from build123d import *

# Parameters (mm, degrees)
BOSS_EXTRUDE2_DEPTH      = 0.79375
FILLET2_R                = 0.396875
CIRPATTERN5_COUNT        = 4
FILLET2_OF_CIRPATTERN5_R = 0.396875
SKETCH6_R                = 10.9855
SKETCH6_R_2              = 9.398
BOSS_EXTRUDE3_DEPTH      = 9.017
SKETCH8_W                = 3.175
SKETCH8_H                = 14.859
SKETCH8_H_2              = 3.175
CUT_EXTRUDE1_DEPTH       = 129.426706448
CUT_EXTRUDE2_REACH       = 130.427
CUT_EXTRUDE2_END_RADIUS  = 10.9855
SKETCH8_3_W              = 3.175
SKETCH8_3_H              = 14.859
SKETCH8_3_H_2            = 3.175


with BuildPart() as part:
    # Sketch3 → Revolve2 (revolve)
    with BuildSketch(Plane(origin=(0, 0, 0), x_dir=(0, 0, -1), z_dir=(1, 0, 0)), mode=Mode.PRIVATE) as revolve2_sk:
        with BuildLine():
            Line((57.15, 12.7), (57.15, 9.525))
            Line((57.15, 9.525), (91.893227671, 9.525))
            ThreePointArc((91.893227671, 9.525), (102.982534669, 8.29739345), (113.534829541, 4.674022024))
            ThreePointArc((113.534829541, 4.674022024), (115.069002319, 4.147228765), (116.68125, 3.96875))
            Line((116.68125, 3.96875), (120.65, 3.96875))
            Line((120.65, 3.96875), (120.65, 3.175))
            Line((120.65, 3.175), (122.2375, 3.175))
            Line((122.2375, 3.175), (125.59178364, 6.52928364))
            Line((125.59178364, 6.52928364), (95.25, 10.32569244))
            ThreePointArc((95.25, 10.32569244), (76.236954553, 12.105847936), (57.15, 12.7))
        make_face()
    revolve(revolve2_sk.sketch.rotate(Axis((0, 0, 0), (0, 0, -1)), 90), axis=Axis((0, 0, 0), (0, 0, -1)))

    # Sketch5 → Boss-Extrude2 (add, symmetric)
    with BuildSketch(Plane(origin=(0, 0, 0), x_dir=(0, 0, -1), z_dir=(1, 0, 0))):
        Polygon((125.59178364, 6.27528364), (95.25, 10.07169244), (119.24178364, 18.97528364), (125.59178364, 18.97528364), align=None)
    boss_extrude2 = extrude(amount=BOSS_EXTRUDE2_DEPTH, both=True)

    # Fillet2
    fillet2_edges = [part.edges().sort_by_distance(p)[0] for p in [
        (0.79375, 18.97528364, -122.41678364),
        (-0.79375, 18.97528364, -122.41678364),
        (0.79375, 14.606978185, -107.47086593),
        (-0.79375, 14.606978185, -107.47086593),
    ]]
    fillet(fillet2_edges, radius=FILLET2_R)

    # CirPattern5: Boss-Extrude2 ×4 about axis
    cirpattern5_axis = Axis((0, 0, 0), (0, 0, 1))
    for i in range(1, CIRPATTERN5_COUNT):
        add(boss_extrude2.rotate(cirpattern5_axis, i * 360 / CIRPATTERN5_COUNT))

    # Fillet2 of CirPattern5
    fillet2_of_cirpattern5_edges = [part.edges().sort_by_distance(p)[0] for p in [
        (-18.97528364, 0.79375, -122.41678364),
        (-18.97528364, -0.79375, -122.41678364),
        (-14.606978185, 0.79375, -107.47086593),
        (-14.606978185, -0.79375, -107.47086593),
        (-0.79375, -18.97528364, -122.41678364),
        (0.79375, -18.97528364, -122.41678364),
        (-0.79375, -14.606978185, -107.47086593),
        (0.79375, -14.606978185, -107.47086593),
        (18.97528364, -0.79375, -122.41678364),
        (18.97528364, 0.79375, -122.41678364),
        (14.606978185, -0.79375, -107.47086593),
        (14.606978185, 0.79375, -107.47086593),
    ]]
    fillet(fillet2_of_cirpattern5_edges, radius=FILLET2_OF_CIRPATTERN5_R)

    # Sketch6 → Boss-Extrude3 (add)
    with BuildSketch(Plane.XY.offset(-57.15)):
        Circle(SKETCH6_R)
        Circle(SKETCH6_R_2, mode=Mode.SUBTRACT)
    extrude(amount=BOSS_EXTRUDE3_DEPTH)

    # Sketch8 → Cut-Extrude1 (cut, through all)
    with BuildSketch(Plane(origin=(0, 0, 0), x_dir=(1, 0, 0), z_dir=(0, 1, 0))):
        with Locations((0, 46.5455)):
            Rectangle(SKETCH8_W, SKETCH8_H)
        with Locations((0, 55.5625)):
            Rectangle(SKETCH8_W, SKETCH8_H_2)
        with Locations((3.175, 55.5625)):
            Rectangle(SKETCH8_W, SKETCH8_H_2)
    extrude(amount=-CUT_EXTRUDE1_DEPTH, mode=Mode.SUBTRACT)

    # Cut-Extrude2: up to this cylinder (the profile starts inside it)
    cut_extrude2_end = Plane(origin=(0, 0, -51.054), z_dir=(0, 0, -1)) * Cylinder(CUT_EXTRUDE2_END_RADIUS, 292.842, mode=Mode.PRIVATE)
    # Sketch8<3> → Cut-Extrude2 (cut, up to the surface)
    with BuildSketch(Plane(origin=(0, 0, 0), x_dir=(1, 0, 0), z_dir=(0, 1, 0)), mode=Mode.PRIVATE) as cut_extrude2_sk1:
        with Locations((0, 46.5455)):
            Rectangle(SKETCH8_3_W, SKETCH8_3_H)
    cut_extrude2_tool1 = extrude(cut_extrude2_sk1.sketch, amount=CUT_EXTRUDE2_REACH, mode=Mode.PRIVATE) & cut_extrude2_end
    add(cut_extrude2_tool1.solids().sort_by_distance((0, 0, -46.5455))[0], mode=Mode.SUBTRACT)
    # Sketch8<3> → Cut-Extrude2 (cut, up to the surface)
    with BuildSketch(Plane(origin=(0, 0, 0), x_dir=(1, 0, 0), z_dir=(0, 1, 0)), mode=Mode.PRIVATE) as cut_extrude2_sk2:
        with Locations((0, 55.5625)):
            Rectangle(SKETCH8_3_W, SKETCH8_3_H_2)
    cut_extrude2_tool2 = extrude(cut_extrude2_sk2.sketch, amount=CUT_EXTRUDE2_REACH, mode=Mode.PRIVATE) & cut_extrude2_end
    add(cut_extrude2_tool2.solids().sort_by_distance((0, 0, -55.5625))[0], mode=Mode.SUBTRACT)
    # Sketch8<3> → Cut-Extrude2 (cut, up to the surface)
    with BuildSketch(Plane(origin=(0, 0, 0), x_dir=(1, 0, 0), z_dir=(0, 1, 0)), mode=Mode.PRIVATE) as cut_extrude2_sk3:
        with Locations((-3.175, 55.5625)):
            Rectangle(SKETCH8_3_W, SKETCH8_3_H_2)
    cut_extrude2_tool3 = extrude(cut_extrude2_sk3.sketch, amount=CUT_EXTRUDE2_REACH, mode=Mode.PRIVATE) & cut_extrude2_end
    add(cut_extrude2_tool3.solids().sort_by_distance((-3.175, 0, -55.5625))[0], mode=Mode.SUBTRACT)


solid = part.part
Geometry: final body of the model. Coordinates: model frame, mm. A direction names the side the tool comes from. Give positions to 0.01 mm unless a question says otherwise; leave off trailing zeros. Use CSV: the item, a comma, the result in double quotes.
1. Contact query for flat-ended pins moving along their axis: pin 1 (3.5 mm diameter, centred on y = -12, z = -108, fed in from -X); pin 2 (1.3 mm diameter, centred on y = -9.5, z = -53, fed in from +X); pin 3 (1.4 mm diameter, centred on y = 9, z = -55, fed in from +X). Output: stop coordinate, or through.
Answers below:
pin 1,"x = -0.79"
pin 2,"x = 6.51"
pin 3,"x = 7.2"
2. Material intervals for line 1 along Y through (x, z) = (0, -121.45) (3 decimals); line 2 along X through (y, z) = (10, -100); line 3 along Y through (x, z) = (4.5, -64), sorted ascending. Write a range as from..to.
Answers below:
line 1,"-18.975..-3.175, 3.175..18.975"
line 2,"-0.79..0.79"
line 3,"-11.79..-8.39, 8.39..11.79"
3. Mould query, pull axis Z, two halves, no side actions, for faces 6 (the face through (-2, -3, -120.65)), 7 (the face through (14.555, -0.006, -107.33)), 8 (the face through (0, 13, -125.592)). Classes: +Z half, -Z half, draft (parallel to the pull), parting line (faces both ways), or undercut.
Answers below:
face 6,"+Z half"
face 7,"undercut"
face 8,"-Z half"
4. Access query for faces 1 (the face through (0.794, -13, -115)), 2 (the face through (-1.588, -10, -53)), 3 (the face through (4.762, -9, -56)), 4 (the face through (-3, 10, -53.975)), 5 (the face through (0.006, 14.555, -107.33)). Directions: +Z, -Z, +X, -X, +Y, -Y. A direction counts if a zero-diameter tool reaches every point of the face in a straight line with its end or side. Return the directions, or none.
Answers below:
face 1,"-Z, +X, -Y"
face 2,"+Z, +Y, -Y"
face 3,"-Y"
face 4,"+Y"
face 5,"+X, -X, +Y"
